Input: dimensioned drawing with shaded views. Units: mm. Origin: part minimum x, y, z. A direction names the side the tool comes from. Round coordinates to 2 decimals unless told otherwise and drop trailing zeros. Order: outer loops, then holes, each group sorted by start corner. A loop starts at its lowest first (then second) coordinate and runs counter-clockwise, first axis right, second up. Notation, with made-up numbers: (57, 23) - (90, 23) arc R31 cw to (90, 59) - close; hole circle Ø5 at (-21, 44). An arc over 180 degrees is marked (long way). Put each result on its own line as item: value. Start each with the question number.
(1) Pin query (flat end, axial travel): P1, Ø5, axis at x = 2.54, y = 2.54, coming from the -Z side; P2, Ø1.5, axis at x = 10, z = 19.5, coming from the +Y side (3 decimals); P3, Ø5, axis at x = 3, z = 18, coming from the +Y side; P4, Ø1.5, axis at y = 11, z = 13.5, coming from the -X side. Return the tip coordinate at first contact, or that it passes through.
(2) Section D-D (x = 10.5). Output: boundary loops of the cut face in (y, z), and give its area (3 significant figures).
(3) Section C-C (z = 6.75). Count the separate pieces of the cut face and the enclosed holes in it, and give its area (3 significant figures).
(4) Section A-A (y = 2.54). Output: boundary loops of the cut face in (x, z), and give its area (3 significant figures).
(5) Pull-direction query (X, two-part tool) for the marked faces 3, 4, 5 and 6; classes: released by +X, released by -X, zero draft, split by the parting line, or undercut.
(6) Material intervals for L1, parallel to Y at x = 2.54, z = 6; L2, parallel to Z at x = 7.75, y = 1; L3, parallel to X at y = 1.5, z = 2, sorted ascending. Write a range as [from, to].
(7) Access query for the marked faces 1 and 2. Directions: +Z, -Z, +X, -X, +Y, -Y. A direction counts if a zero-diameter tool reaches every point of the face in a straight line with its end or side. Return the directions, or none.
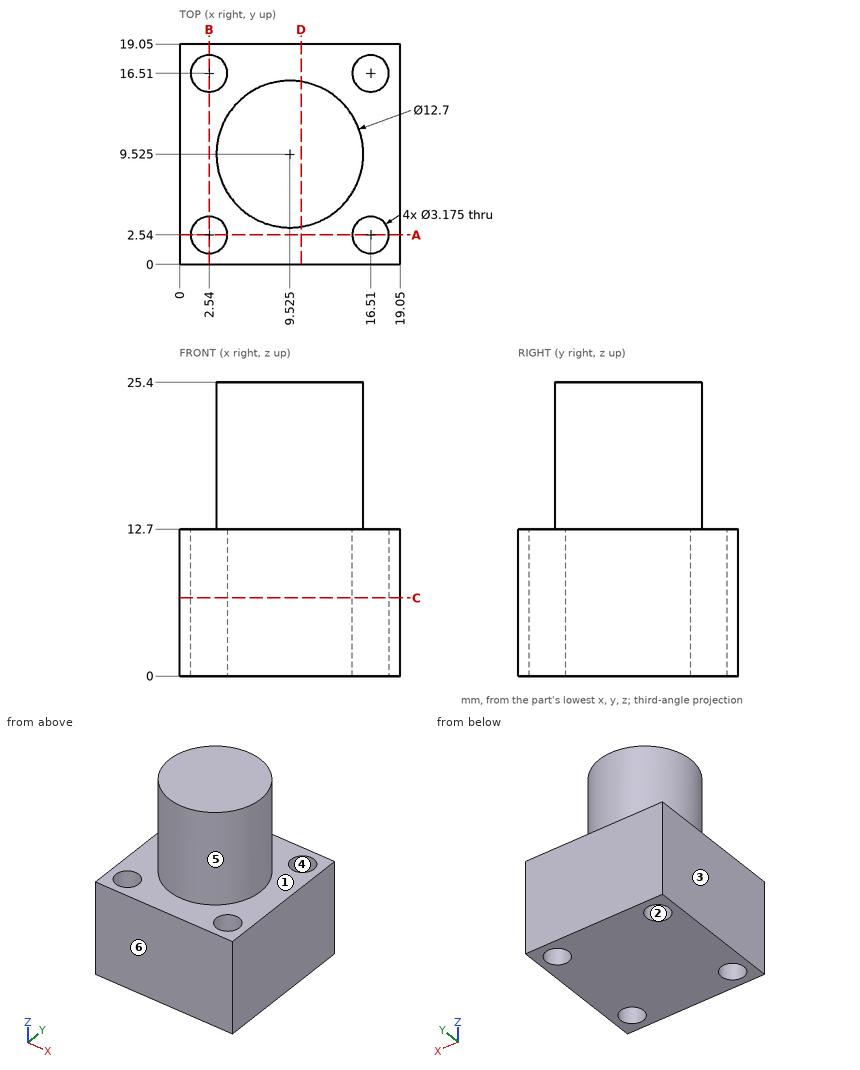
Checks:
1. P1: stops at z = 0
1. P2: stops at y = 15.875
1. P3: stops at y = 14.44
1. P4: stops at x = 3.22
2. outline: (0, 0) - (19.05, 0) - (19.05, 12.7) - (15.8, 12.7) - (15.8, 25.4) - (3.25, 25.4) - (3.25, 12.7) - (0, 12.7) - close
2. area: 401 mm²
3. separate pieces: 1
3. enclosed holes: 4
3. area: 331 mm²
4. outline: (0, 0) - (0.95, 0) - (0.95, 12.7) - (0, 12.7) - close; (4.13, 0) - (14.92, 0) - (14.92, 12.7) - (4.13, 12.7) - close; (18.1, 0) - (19.05, 0) - (19.05, 12.7) - (18.1, 12.7) - close
4. area: 161 mm²
5. face 3: released by -X
5. face 4: undercut
5. face 5: split by the parting line
5. face 6: zero draft
6. L1: y = [0, 0.95], [4.13, 14.92], [18.1, 19.05]
6. L2: z = [0, 12.7]
6. L3: x = [0, 1.34], [3.74, 15.31], [17.71, 19.05]
7. face 1: +Z
7. face 2: +Z, -Z
